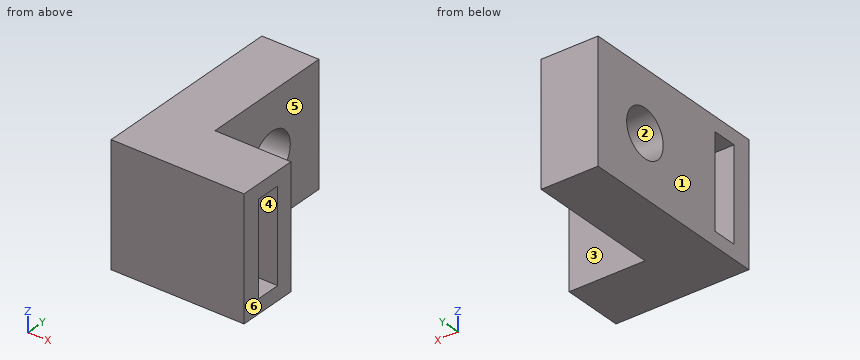
Autodesk Inventor part; units mm, degrees
ref_plane "YZ Plane" through (0, 0, 0) normal (1, 0, 0) x (0, 1, 0)
ref_plane "XZ Plane" through (0, 0, 0) normal (0, 1, 0) x (-1, 0, 0)
ref_plane "XY Plane" through (0, 0, 0) normal (0, 0, 1) x (1, 0, 0)
sketch "Sketch1" plane through (0, 0, 0) normal (1, 0, 0) x (0, 1, 0)
  line L0 (0, 0) -> (25.75, 0)
  line L1 (25.75, 0) -> (25.75, -16)
  line L2 (25.75, -16) -> (0, -16)
  line L3 (0, -16) -> (0, 0)
  line L4 (0, 0) -> (2.5, 0) construction
  line L5 (2.5, 0) -> (2.5, -16) construction
  line L6 (2.5, -16) -> (0, -16) construction
  line L7 (0, -16) -> (0, 0) construction
  line L8 (0, 0) -> (1.875, 0) construction
  line L9 (0, -2.8568) -> (0, 0) construction
  line L10 (0, 0) -> (25.75, 0) construction
  line L11 (25.75, 0) -> (25.75, -1.875) construction
  line L12 (25.75, -1.875) -> (0, -1.875) construction
  line L13 (0, -1.875) -> (0, 0) construction
  line L14 (25.75, -16) -> (0, -16) construction
  line L15 (0, -16) -> (0, -14.125) construction
  line L16 (0, -14.125) -> (25.75, -14.125) construction
  line L17 (25.75, -14.125) -> (25.75, -16) construction
  line L18 (2.5, -1.875) -> (5.75, -1.875)
  line L19 (5.75, -1.875) -> (5.75, -14.125)
  line L20 (5.75, -14.125) -> (2.5, -14.125)
  line L21 (2.5, -14.125) -> (2.5, -1.875)
  circle A0 centre (17.75, -8) radius 3.125
  dimension "d0" = 25.75
  dimension "d1" = 16
  dimension "d2" = 2.5
  dimension "d4" = 1.875
  dimension "d5" = 1.875
  dimension "d6" = 3.25
  dimension "d7" = 6.25
extrude "Extrusion1" add sketch "Sketch1" along normal blind 7.5
sketch "Sketch2" plane through (7.5, 0, 0) normal (1, 0, 0) x (0, 0, -1)
  line L0 (0, 0) -> (16, 0)
  line L1 (16, 0) -> (16, 25.75)
  line L2 (0, 0) -> (16, 0)
  line L3 (16, 0) -> (16, 8)
  line L4 (16, 8) -> (0, 8)
  line L5 (0, 8) -> (0, 0)
  line L6 (1.875, 2.5) -> (1.875, 5.75)
  line L7 (14.125, 5.75) -> (14.125, 2.5)
  line L8 (1.875, 5.75) -> (14.125, 5.75)
  line L9 (14.125, 5.75) -> (14.125, 2.5)
  line L10 (14.125, 2.5) -> (1.875, 2.5)
  line L11 (1.875, 2.5) -> (1.875, 5.75)
  dimension "d10" = 8
extrude "Extrusion2" add sketch "Sketch2" along normal blind 10
properties part number "_3DPrint"
The listing builds one solid part. Answer for the finished solid, in the listing's coordinates (mm). Face numbers are marked on the shaded views. A direction names the side the tool comes from. Give positions to 0.01 mm unless a question says otherwise; leave off trailing zeros. Write each loop counter-clockwise with the first axis right and the second up, starting at its lowest first coordinate (ties: lowest second). Pieces come first, ordered by that corner, then holes. Notation, with made-up numbers: (35, -10) - (84, -10) arc R30 ccw to (84, 29) - close; hole circle Ø4 at (32, 69.5). An arc over 180 degrees is marked (long way). Use a Markdown table: item, result.
1. Each of these flat-tipped pins is pushed along its axis until it touches: P1, Ø1, axis at x = 7, z = -13.5, coming from the -Y side; P2, Ø8, axis at x = 12, z = -5.5, coming from the +Y side; P3, Ø1.5, axis at y = 18, z = -11, coming from the +X side; P4, Ø4, axis at y = 17.75, z = -8, coming from the -X side. Where does it stop, or does it pass through?
Values follow:
| item | result |
|---|---|
| P1 | stops at y = 0 |
| P2 | stops at y = 8 |
| P3 | stops at x = 7.5 |
| P4 | passes through |
2. Section D-D on x = 6 is taken. Write down the section's boundary in (y, z) (3 decimals), plus the area to 3 significant figures.
Values follow:
| item | result |
|---|---|
| outline | (0, -16) - (25.75, -16) - (25.75, 0) - (0, 0) - close; hole (2.5, -14.125) - (5.75, -14.125) - (5.75, -1.875) - (2.5, -1.875) - close; hole circle Ø6.25 at (17.75, -8) |
| area | 342 mm² |
3. Section B-B on y = 17.75 is taken. Write down the section's boundary in (x, z) (3 decimals).
Values follow:
| item | result |
|---|---|
| outline | (0, -16) - (7.5, -16) - (7.5, -11.125) - (0, -11.125) - close; (0, -4.875) - (7.5, -4.875) - (7.5, 0) - (0, 0) - close |
4. Section C-C on z = -12.75 is taken. Write down the section's boundary in (x, y).
Values follow:
| item | result |
|---|---|
| outline | (0, 0) - (17.5, 0) - (17.5, 2.5) - (0, 2.5) - close; (0, 5.75) - (17.5, 5.75) - (17.5, 8) - (7.5, 8) - (7.5, 25.75) - (0, 25.75) - close |
5. Find the intervals of material crossed by probe 1 along Y at (x, z) = (16, -7); probe 2 along Z at (x, y) = (6.25, 17.75) (3 decimals); probe 3 along Y at (x, z) = (4, -6.75), in increasing order. Write a range as from..to.
Values follow:
| item | result |
|---|---|
| probe 1 | y = 0..2.5, 5.75..8 |
| probe 2 | z = -16..-11.125, -4.875..0 |
| probe 3 | y = 0..2.5, 5.75..14.89, 20.61..25.75 |
6. Section A-A on z = -8 is taken. Write down the section's boundary in (x, y) (3 decimals), plus the area to 3 significant figures.
Values follow:
| item | result |
|---|---|
| outline | (0, 0) - (17.5, 0) - (17.5, 2.5) - (0, 2.5) - close; (0, 5.75) - (17.5, 5.75) - (17.5, 8) - (7.5, 8) - (7.5, 14.625) - (0, 14.625) - close; (0, 20.875) - (7.5, 20.875) - (7.5, 25.75) - (0, 25.75) - close |
| area | 169 mm² |
7. For a pull along Y with two mould halves and no side action, classify the marked faces 1, 2 and 3 as released by +Y, released by -Y, zero draft, split by the parting line, or undercut.
Values follow:
| item | result |
|---|---|
| face 1 | zero draft |
| face 2 | undercut |
| face 3 | released by +Y |
8. A tool of negligible diameter and unlimited length cuts with its end or side. For the marked faces 4, 5 and 6, from which of +Z, -Z, +X, -X, +Y, -Y can it reach the whole face along a straight path? Write none if from no direction.
Values follow:
| item | result |
|---|---|
| face 4 | +X, -X |
| face 5 | +Z, -Z, +X, +Y |
| face 6 | +Z, -Z, +X, +Y, -Y |
